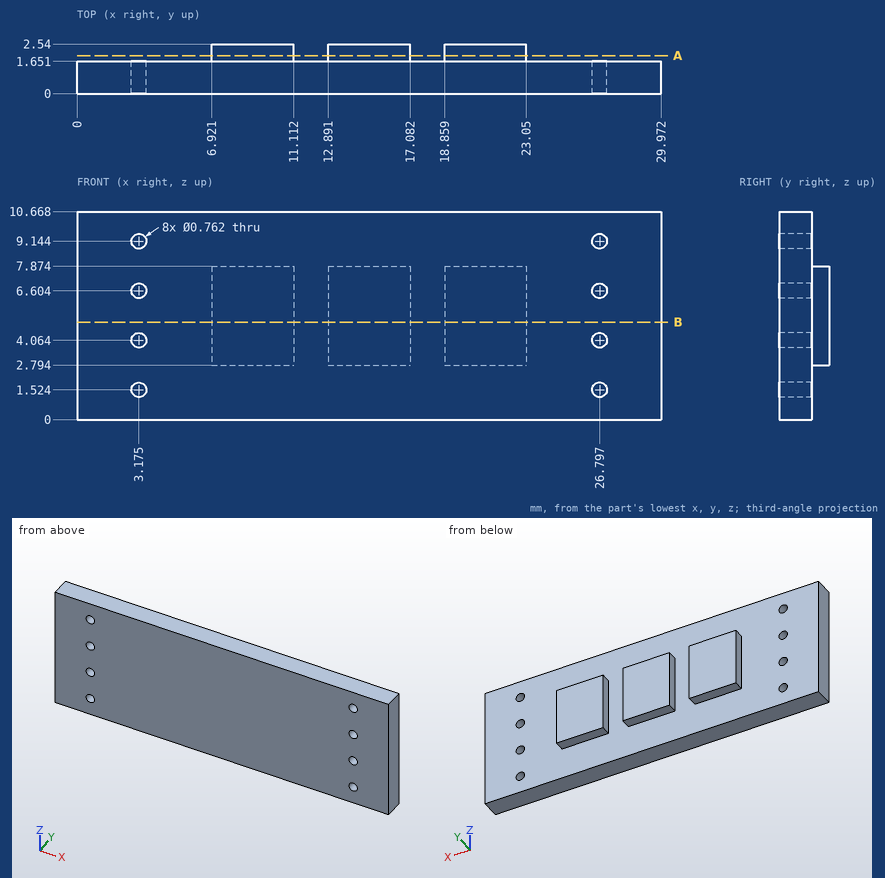
Source: three-view drawing plus pictorial views. Frame: mm from the lowest corner of the part. Give positions to 0.01 mm unless a question says otherwise; leave off trailing zeros. Order: outer loops, then holes, each group sorted by start corner. A loop starts at its lowest first (then second) coordinate and runs counter-clockwise, first axis right, second up. Notation, with made-up numbers: (37.5, -38.5) -> (55.5, -38.5) arc R14 cw to (55.5, -16.5) -> close; hole circle Ø10 at (43.25, 56). An arc over 180 degrees is marked (long way). Write each question's results on one line, items separated by ' | '. Start each with the question number.
Item 1: Contact query for a flat-ended pin moving along its axis: P1, Ø0.7, axis at x = 15, y = 2.5, coming from the +Z side. Output: stop coordinate, or through.
Item 2: Cut plane B-B on z = 5. Return the cut outline in (x, y).
Item 3: Line query: line 1 (X direction, y = 2.1, z = 7.5); line 2 (Y direction, x = 16, z = 9); line 3 (X direction, y = 0.6, z = 6.5) (1 decimal). Output: solid intervals per line, ascending.
Item 4: Cut plane A-A on y = 1.95. Give the number of separate pieces and of enclosed holes in the cut face.
Established:
1) P1: z = 7.87
2) outline: (0, 0) -> (29.97, 0) -> (29.97, 1.65) -> (23.05, 1.65) -> (23.05, 2.54) -> (18.86, 2.54) -> (18.86, 1.65) -> (17.08, 1.65) -> (17.08, 2.54) -> (12.89, 2.54) -> (12.89, 1.65) -> (11.11, 1.65) -> (11.11, 2.54) -> (6.92, 2.54) -> (6.92, 1.65) -> (0, 1.65) -> close
3) line 1: 6.92 to 11.11, 12.89 to 17.08, 18.86 to 23.05 | line 2: 0 to 1.65 | line 3: 0 to 2.8, 3.5 to 26.4, 27.2 to 30
4) separate pieces: 3 | enclosed holes: 0
